Autodesk Inventor part; units mm, degrees
ref_plane "YZ Plane" through (0, 0, 0) normal (1, 0, 0) x (0, 1, 0)
ref_plane "XZ Plane" through (0, 0, 0) normal (0, 1, 0) x (-1, 0, 0)
ref_plane "XY Plane" through (0, 0, 0) normal (0, 0, 1) x (1, 0, 0)
sketch "Sketch1" plane through (0, 0, 0) normal (0, 0, 1) x (1, 0, 0)
  line L0 (3.175, 0) -> (22.225, 0)
  line L1 (25.4, 3.175) -> (25.4, 22.225)
  line L2 (22.225, 25.4) -> (3.175, 25.4)
  line L3 (0, 22.225) -> (0, 3.175)
  arc A0 (3.175, 25.4) -> (0, 22.225) centre (3.175, 22.225) ccw
  arc A1 (25.4, 22.225) -> (22.225, 25.4) centre (22.225, 22.225) ccw
  arc A2 (22.225, 0) -> (25.4, 3.175) centre (22.225, 3.175) ccw
  arc A3 (0, 3.175) -> (3.175, 0) centre (3.175, 3.175) ccw
  line L4 (6.35, 3.175) -> (19.05, 3.175)
  line L5 (22.225, 6.35) -> (22.225, 19.05)
  line L6 (19.05, 22.225) -> (6.35, 22.225)
  line L7 (3.175, 19.05) -> (3.175, 6.35)
  arc A4 (6.35, 22.225) -> (3.175, 19.05) centre (6.35, 19.05) ccw
  arc A5 (19.05, 3.175) -> (22.225, 6.35) centre (19.05, 6.35) ccw
  arc A6 (22.225, 19.05) -> (19.05, 22.225) centre (19.05, 19.05) ccw
  arc A7 (3.175, 6.35) -> (6.35, 3.175) centre (6.35, 6.35) ccw
  point P0 (0, 0)
  point P1 (25.4, 25.4)
  point P2 (25.4, 0)
  point P3 (0, 25.4)
  dimension "d0" = 25.4
  dimension "d1" = 25.4
  dimension "d2" = 3.175
  dimension "d3" = 3.175
extrude "Extrusion1" add sketch "Sketch1" along normal blind 304.8
properties part number "SteelPipe12in"
Design review of the part built by this model. Coordinates are the model's own, in mm. A direction names the side the tool comes from. Coordinates: 2 decimals unless noted, no trailing zeros. Write each loop counter-clockwise with the first axis right and the second up, starting at its lowest first coordinate (ties: lowest second). Pieces come first, ordered by that corner, then holes. Notation, with made-up numbers: (26.25, -35.5) -> (53.25, -35.5) arc R32 cw to (53.25, -5.5) -> close; hole circle Ø3 at (-27.5, 14.25). An arc over 180 degrees is marked (long way). Write each question's results on one line, items separated by ' | '. Start each with the question number.
(1) Take a section at C-C on z = 159. Write out the cut boundary in (x, y) (3 decimals), and give its area (3 significant figures).
(2) Take a section at A-A on y = 15.25. Write out the cut boundary in (x, z) (3 decimals).
(3) Tool access review of faces 5 (the face through (13, 3.175, 150)), 6 (the face through (13, 0, 150)): name each direction out of +Z, -Z, +X, -X, +Y, -Y from which nothing blocks a thin tool from reaching the whole face with its end or side.
(4) The part is to be moulded in two halves that separate along X. For faces 1 (the face through (0, 13, 150)), 2 (the face through (13, 22.225, 150)), 3 (the face through (3.175, 13, 150)), 4 (the face through (1, 13, 0)), say which applies: pulls with the +X half, pulls with the -X half, needs draft (parallel to the pull), parting line crosses it, or undercut.
(5) For line 1 along Y through (x, z) = (6, 151); line 2 along X through (y, z) = (7.75, 48.5) (3 decimals); line 3 along Y through (x, z) = (21.75, 186), list the stretches that pass through material, from the lowest coordinate up. Write a range as from..to.
Results found:
1) outline: (0, 3.175) arc R3.175 ccw to (3.175, 0) -> (22.225, 0) arc R3.175 ccw to (25.4, 3.175) -> (25.4, 22.225) arc R3.175 ccw to (22.225, 25.4) -> (3.175, 25.4) arc R3.175 ccw to (0, 22.225) -> close; hole (3.175, 6.35) arc R3.175 ccw to (6.35, 3.175) -> (19.05, 3.175) arc R3.175 ccw to (22.225, 6.35) -> (22.225, 19.05) arc R3.175 ccw to (19.05, 22.225) -> (6.35, 22.225) arc R3.175 ccw to (3.175, 19.05) -> close | area: 282 mm2
2) outline: (0, 0) -> (3.175, 0) -> (3.175, 304.8) -> (0, 304.8) -> close; (22.225, 0) -> (25.4, 0) -> (25.4, 304.8) -> (22.225, 304.8) -> close
3) face 5: +Z, -Z | face 6: +Z, -Z, +X, -X, -Y
4) face 1: pulls with the -X half | face 2: undercut | face 3: undercut | face 4: needs draft
5) line 1: y = 0..3.19, 22.21..25.4 | line 2: x = 0..3.175, 22.225..25.4 | line 3: y = 0..4.68, 20.72..25.4
